Build history of the part. All positions in model axes, mm. Give positions to 0.01 mm unless a question says otherwise; leave off trailing zeros. Write each loop counter-clockwise with the first axis right and the second up, starting at its lowest first coordinate (ties: lowest second). Pieces come first, ordered by that corner, then holes.
from build123d import *

# Parameters (mm, degrees)
F0_R      = 3
F0_R_2    = 5
F1_DEPTH  = 5
F1_FACE_W = 100
F1_FACE_H = 5
F2_DEPTH  = 2
F3_DEPTH  = 5


with BuildPart() as f1:
    # F0 (on Front) → F1 (new body)
    with BuildSketch(Plane.XZ):
        Polygon((-80.611844, -2.364473), (31.388156, -2.364473), (19.388156, 25.835527), (-80.611844, 25.835527), align=None)
        with Locations((-38.611844, 2.635527)):
            Circle(F0_R, mode=Mode.SUBTRACT)
        with Locations((-8.611844, 2.635527)):
            Circle(F0_R, mode=Mode.SUBTRACT)
        with Locations((21.388156, 2.635527)):
            Circle(F0_R, mode=Mode.SUBTRACT)
        with Locations((-60.611844, 15.835527)):
            Circle(F0_R_2, mode=Mode.SUBTRACT)
    extrude(amount=F1_DEPTH)

    # F1_face (on face) → F2 (cut)
    with BuildSketch(Plane(origin=(-30.611844, -2.5, 25.835527), x_dir=(1, 0, 0), z_dir=(0, 0, 1))):
        Rectangle(F1_FACE_W, F1_FACE_H)
    extrude(amount=-F2_DEPTH, mode=Mode.SUBTRACT)

    # F0 (on Front) → F3 (join)
    with BuildSketch(Plane.XZ):
        Polygon((-80.611844, -2.364473), (31.388156, -2.364473), (19.388156, 25.835527), (-80.611844, 25.835527), align=None)
        with Locations((-38.611844, 2.635527)):
            Circle(F0_R, mode=Mode.SUBTRACT)
        with Locations((-8.611844, 2.635527)):
            Circle(F0_R, mode=Mode.SUBTRACT)
        with Locations((21.388156, 2.635527)):
            Circle(F0_R, mode=Mode.SUBTRACT)
        with Locations((-60.611844, 15.835527)):
            Circle(F0_R_2, mode=Mode.SUBTRACT)
    extrude(amount=F3_DEPTH)


solid = f1.part
1. Mould opens along X. For faces 1 (the face through (-5.75, -2.46, 3.54)), 2 (the face through (-25, -5, 12)), 3 (the face through (-80.612, -2, 12)) say: pulls with the +X half, pulls with the -X half, needs draft (parallel to the pull), parting line crosses it, or undercut.
2. Saw through at C-C on z = 4.25. Give the cut face in (x, y), plus the area to 3 significant figures.
3. Saw through at A-A on z = 14.75. Give the cut face in (x, y), plus the area to 3 significant figures.
4. Saw through at B-B on y = -0.75. Give the cut face in (x, z).
5. Drill centre lines: line 1 along X through (y, z) = (-0.4, 3); line 2 along X through (y, z) = (-4.35, 0); line 3 along Z through (x, y) = (-7, -3.3). Where is each one in solid material? Low to high.
6. Drop flat-ended pins along their axis: pin 1 (2 mm diameter, centred on y = -1, z = 21.5, fed in from +X); pin 2 (10 mm diameter, centred on x = -39.5, z = 3.5, fed in from -Y); pin 3 (1.5 mm diameter, centred on y = -3.5, z = 2.5, fed in from +X). Give the stop position or say it passes through.
Outcome:
1. face 1: undercut
1. face 2: needs draft
1. face 3: pulls with the -X half
2. outline: (-80.61, -5) - (-41.14, -5) - (-41.14, 0) - (-80.61, 0) - close; (-36.08, -5) - (-11.14, -5) - (-11.14, 0) - (-36.08, 0) - close; (-6.08, -5) - (18.86, -5) - (18.86, 0) - (-6.08, 0) - close; (23.92, -5) - (28.57, -5) - (28.57, 0) - (23.92, 0) - close
2. area: 470 mm2
3. outline: (-80.61, -5) - (-65.49, -5) - (-65.49, 0) - (-80.61, 0) - close; (-55.73, -5) - (24.11, -5) - (24.11, 0) - (-55.73, 0) - close
3. area: 475 mm2
4. outline: (-80.61, -2.36) - (31.39, -2.36) - (19.39, 25.84) - (-80.61, 25.84) - close; hole circle Ø10 at (-60.61, 15.84); hole circle Ø6 at (-38.61, 2.64); hole circle Ø6 at (-8.61, 2.64); hole circle Ø6 at (21.39, 2.64)
5. line 1: x = -80.61 to -41.59, -35.63 to -11.59, -5.63 to 18.41, 24.37 to 29.11
5. line 2: x = -80.61 to -40.05, -37.18 to -10.05, -7.18 to 19.95, 22.82 to 30.38
5. line 3: z = -2.36 to 0.11, 5.17 to 25.84
6. pin 1: stops at x = 21.66
6. pin 2: stops at y = -5
6. pin 3: stops at x = 29.64
